Geometry: see drawing. Coordinates: mm, zero at the bounding-box minimum. Round coordinates to 2 decimals unless told otherwise and drop trailing zeros. Loops run counter-clockwise (first coordinate to the right, second up) from the corner with the lowest first, then second, coordinate; pieces in that order, holes last. Notation, with made-up numbers: (16, 71.25) - (75, 71.25) arc R27 cw to (75, 101.25) - close; hole circle Ø11 at (51, 21). An arc over 180 degrees is marked (long way). Return JSON: item names as keys, results as strings. Group by question number.
1. First-contact query: pin 1 Ø2 at (x, y) = (2, 4) entering from -Z. Flat tip, straight axial feed; report the tip coordinate or a pass-through.
2. Section A-A on z = 0.1. Return loops of the section in (x, y).
3. Material intervals for probe 1 along Y at (x, z) = (7, 0.3); probe 2 along X at (y, z) = (2.5, 0.5); probe 3 along X at (y, z) = (1.5, 0.25), sorted ascending.
4. Section B-B on x = 6.5. Return loops of the section in (y, z).
5. Section C-C on y = 4. Return loops of the section in (x, z).
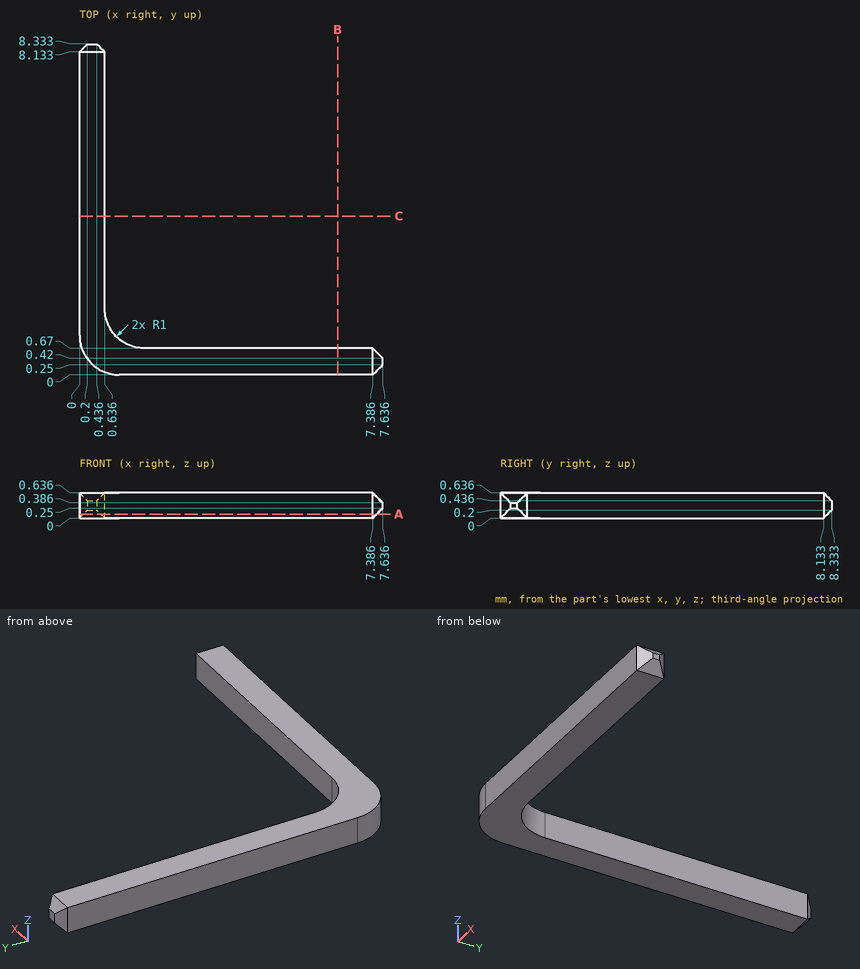
Taken from the geometry:
{
 "1": {"pin 1": "through"},
 "2": {"outline": "(0, 1) arc R1 ccw to (1, 0) - (7.39, 0) - (7.49, 0.1) - (7.49, 0.57) - (7.39, 0.67) - (1.64, 0.67) arc R1 cw to (0.64, 1.67) - (0.64, 8.13) - (0.54, 8.23) - (0.1, 8.23) - (0, 8.13) - close"},
 "3": {"probe 1": "0 to 0.67", "probe 2": "0 to 0.64", "probe 3": "0 to 0.65"},
 "4": {"outline": "(0, 0) - (0.67, 0) - (0.67, 0.64) - (0, 0.64) - close"},
 "5": {"outline": "(0, 0) - (0.64, 0) - (0.64, 0.64) - (0, 0.64) - close"}
}
